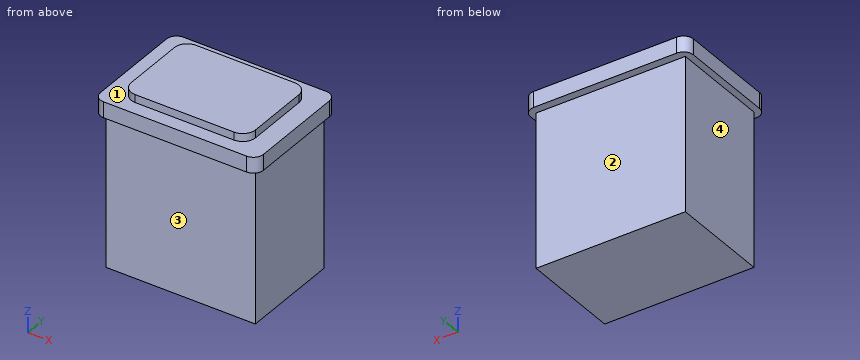
Solid Edge part; units mm, degrees
sketch "Sketch1" plane through (0, 0, 0) normal (0, 0, 1) x (1, 0, 0)
  line L0 (10.4775, 7.493) -> (-10.4775, 7.493)
  line L1 (-10.4775, 7.493) -> (-10.4775, -7.493)
  line L2 (-10.4775, -7.493) -> (10.4775, -7.493)
  line L3 (10.4775, -7.493) -> (10.4775, 7.493)
extrude "Protrusion1" add sketch "Sketch1" along normal blind 2.032
sketch "Sketch2" plane through (0, 0, 0) normal (0, 0, 1) x (1, 0, 0)
  line L0 (9.6012, -6.4516) -> (9.6012, 6.4516)
  line L1 (9.6012, 6.4516) -> (-9.6012, 6.4516)
  line L2 (-9.6012, 6.4516) -> (-9.6012, -6.4516)
  line L3 (-9.6012, -6.4516) -> (9.6012, -6.4516)
extrude "ExtrudedProtrusion_2" add sketch "Sketch2" against normal blind 19.812
sketch "Sketch3" plane through (0, 0, 0) normal (0, 0, 1) x (1, 0, 0)
  line L0 (8.001, -5.715) -> (8.001, 5.715)
  line L1 (8.001, 5.715) -> (-8.001, 5.715)
  line L2 (-8.001, 5.715) -> (-8.001, -5.715)
  line L3 (-8.001, -5.715) -> (8.001, -5.715)
extrude "ExtrudedProtrusion_3" add sketch "Sketch3" along normal blind 3.048
fillet "Round_1" radius 1.27 4 edges at (-10.4775, 7.493, 1.016) (-10.4775, -7.493, 1.016) (10.4775, 7.493, 1.016) (10.4775, -7.493, 1.016)
fillet "Round_2" radius 1.651 4 edges at (8.001, -5.715, 2.54) (8.001, 5.715, 2.54) (-8.001, -5.715, 2.54) (-8.001, 5.715, 2.54)
Geometry check sheet. Reference: the model listing, model coordinates, mm. Face numbers are marked on the shaded views. A direction names the side the tool comes from. Round coordinates to 2 decimals unless told otherwise and drop trailing zeros. Loops run counter-clockwise (first coordinate to the right, second up) from the corner with the lowest first, then second, coordinate; pieces in that order, holes last.
Item 1: Cross-section at A-A on x = -8.75. Record the boundary of the cut face in (y, z), then the cut area to 3 significant figures.
Item 2: Cross-section at D-D on x = 4. Record the boundary of the cut face in (y, z) (3 decimals), then the cut area to 3 significant figures.
Item 3: Gauge pin test, flat ends, axial feed: pin 1 (8 mm diameter, centred on y = -2.5, z = -7.5, fed in from -X); pin 2 (1.1 mm diameter, centred on x = 0, z = 3, fed in from +Y) (3 decimals); pin 3 (6.5 mm diameter, centred on y = 1, z = -7, fed in from +X). Record the tip position at first contact, or that the pin passes through.
Item 4: Access from +Z, -Z, +X, -X, +Y, -Y to the whole of each face (thin tool, end or side, straight path). Record for the marked faces 1, 2, 3 and 4.
Item 5: Cross-section at B-B on y = -2.75. Record the boundary of the cut face in (x, z), then the cut area to 3 significant figures.
Item 6: Cross-section at C-C on z = -2. Record the boundary of the cut face in (x, y), then the cut area to 3 significant figures.
Item 7: Thickness scan on line 1 (Z direction, x = -7, y = 6); line 2 (X direction, y = -1.75, z = -4); line 3 (Y direction, x = 3.5, z = -0.5). Record the ranges inside material, lowest first.
Answer sheet:
1. outline: (-7.49, 0) - (-6.45, 0) - (-6.45, -19.81) - (6.45, -19.81) - (6.45, 0) - (7.49, 0) - (7.49, 2.03) - (-7.49, 2.03) - close
1. area: 286 mm2
2. outline: (-7.493, 0) - (-6.452, 0) - (-6.452, -19.812) - (6.452, -19.812) - (6.452, 0) - (7.493, 0) - (7.493, 2.032) - (5.715, 2.032) - (5.715, 3.048) - (-5.715, 3.048) - (-5.715, 2.032) - (-7.493, 2.032) - close
2. area: 298 mm2
3. pin 1: stops at x = -9.6
3. pin 2: stops at y = 5.715
3. pin 3: stops at x = 9.6
4. face 1: +Z
4. face 2: -Z, +X, -X, +Y
4. face 3: -Z, +X, -X, -Y
4. face 4: -Z, -X, +Y, -Y
5. outline: (-10.48, 0) - (-9.6, 0) - (-9.6, -19.81) - (9.6, -19.81) - (9.6, 0) - (10.48, 0) - (10.48, 2.03) - (8, 2.03) - (8, 3.05) - (-8, 3.05) - (-8, 2.03) - (-10.48, 2.03) - close
5. area: 439 mm2
6. outline: (-9.6, -6.45) - (9.6, -6.45) - (9.6, 6.45) - (-9.6, 6.45) - close
6. area: 248 mm2
7. line 1: z = -19.81 to 2.03
7. line 2: x = -9.6 to 9.6
7. line 3: y = -6.45 to 6.45
